Build history of the part. All positions in model axes, mm. Round coordinates to 2 decimals unless told otherwise and drop trailing zeros. Write each loop counter-clockwise with the first axis right and the second up, starting at its lowest first coordinate (ties: lowest second). Pieces come first, ordered by that corner, then holes.
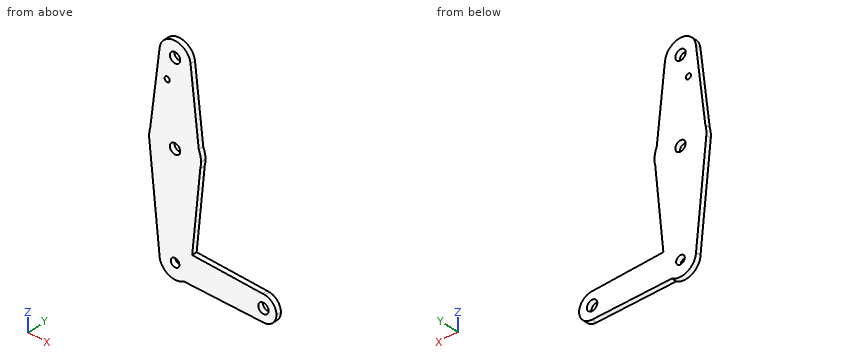
from build123d import *

# Parameters (mm, degrees)
F0_R     = 3.175
F0_R_2   = 2.6335759293
F0_R_3   = 1.5875
F1_DEPTH = 3.048


with BuildPart() as f1:
    # F0 (on Front) → F1 (new body)
    with BuildSketch(Plane.XZ):
        with BuildLine():
            ThreePointArc((56.7990275078, -24.9062731053), (62.4116875835, -22.581433181), (64.7365275078, -16.9687731053))
            ThreePointArc((64.7365275078, -16.9687731053), (62.7426623776, -11.707869116), (57.7627673101, -9.0899970681))
            Line((57.7627673101, -9.0899970681), (56.297547037, -9.0471303724))
            ThreePointArc((56.297547037, -9.0471303724), (48.8654928151, -17.2196386647), (56.7990275078, -24.9062731053))
        make_face()
        with Locations((56.7990275078, -16.9687731053)):
            Circle(F0_R, mode=Mode.SUBTRACT)
        with BuildLine():
            Line((56.297547037, -9.0471303724), (57.7627673101, -9.0899970681))
            ThreePointArc((57.7627673101, -9.0899970681), (57.0311488355, -9.0346678666), (56.297547037, -9.0471303724))
        make_face()
        with BuildLine():
            Line((8.0107625365, -24.9062731053), (56.7990275078, -24.9062731053))
            ThreePointArc((56.7990275078, -24.9062731053), (48.8654928151, -17.2196386647), (56.297547037, -9.0471303724))
            Line((56.297547037, -9.0471303724), (13.2168797338, -7.7867561536))
            Line((13.2168797338, -7.7867561536), (12.2251364065, -17.8985078123))
            ThreePointArc((12.2251364065, -17.8985078123), (10.9082443644, -21.8776629611), (8.0107625365, -24.9062731053))
        make_face()
        with BuildLine():
            ThreePointArc((-6.7763501221, -17.208975122), (-1.652361496, -25.4176415362), (8.0107625365, -24.9062731053))
            ThreePointArc((8.0107625365, -24.9062731053), (10.9082443644, -21.8776629611), (12.2251364065, -17.8985078123))
            ThreePointArc((12.2251364065, -17.8985078123), (12.2592428174, -17.4341964193), (12.2706206818, -16.9687731053))
            ThreePointArc((12.2706206818, -16.9687731053), (9.8779825256, -10.6556883181), (3.9021084446, -7.5142418607))
            ThreePointArc((3.9021084446, -7.5142418607), (-3.6569014681, -9.9165865564), (-6.7763501221, -17.208975122))
        make_face()
        with Locations((2.7456206818, -16.9687731053)):
            Circle(F0_R_2, mode=Mode.SUBTRACT)
        with BuildLine():
            Line((3.9021084446, -7.5142418607), (13.2168797338, -7.7867561536))
            Line((13.2168797338, -7.7867561536), (18.1800145925, 42.8170500531))
            ThreePointArc((18.1800145925, 42.8170500531), (1.6704584717, 30.6926773645), (-13.0491238986, 44.9369657372))
            Line((-13.0491238986, 44.9369657372), (-6.7763501221, -17.208975122))
            ThreePointArc((-6.7763501221, -17.208975122), (-3.6569014681, -9.9165865564), (3.9021084446, -7.5142418607))
        make_face()
        with BuildLine():
            Line((12.2251364065, -17.8985078123), (13.2168797338, -7.7867561536))
            Line((13.2168797338, -7.7867561536), (3.9021084446, -7.5142418607))
            ThreePointArc((3.9021084446, -7.5142418607), (9.8779825256, -10.6556883181), (12.2706206818, -16.9687731053))
            ThreePointArc((12.2706206818, -16.9687731053), (12.2592428174, -17.4341964193), (12.2251364065, -17.8985078123))
        make_face()
        with BuildLine():
            ThreePointArc((-13.0491238986, 44.9369657372), (1.6704584717, 30.6926773645), (18.1800145925, 42.8170500531))
            ThreePointArc((18.1800145925, 42.8170500531), (18.5100843316, 44.6611170492), (18.6206206818, 46.5312268947))
            ThreePointArc((18.6206206818, 46.5312268947), (18.2740618453, 49.830187342), (17.2495164257, 52.9851120231))
            ThreePointArc((17.2495164257, 52.9851120231), (1.7136407932, 62.3726486273), (-12.4730077607, 51.0488560659))
            ThreePointArc((-12.4730077607, 51.0488560659), (-13.0593192868, 48.0210247289), (-13.0491238986, 44.9369657372))
        make_face()
        with Locations((2.7456206818, 46.5312268947)):
            Circle(F0_R, mode=Mode.SUBTRACT)
        with BuildLine():
            Line((-6.7441452961, 98.1497418202), (-12.4730077607, 51.0488560659))
            ThreePointArc((-12.4730077607, 51.0488560659), (1.7136407932, 62.3726486273), (17.2495164257, 52.9851120231))
            Line((17.2495164257, 52.9851120231), (12.2125248757, 98.3816315712))
            ThreePointArc((12.2125248757, 98.3816315712), (12.2560856402, 97.8572319106), (12.2706206818, 97.3312268947))
            ThreePointArc((12.2706206818, 97.3312268947), (2.3359842212, 87.8150394769), (-6.7441452961, 98.1497418202))
        make_face()
        with Locations((-2.1043515299, 83.0673798919)):
            Circle(F0_R_3, mode=Mode.SUBTRACT)
        with BuildLine():
            ThreePointArc((12.2125248757, 98.3816315712), (2.6291136887, 106.8555143284), (-6.7441452961, 98.1497418202))
            ThreePointArc((-6.7441452961, 98.1497418202), (2.3359842212, 87.8150394769), (12.2706206818, 97.3312268947))
            ThreePointArc((12.2706206818, 97.3312268947), (12.2560856402, 97.8572319106), (12.2125248757, 98.3816315712))
        make_face()
        with Locations((2.7456206818, 97.3312268947)):
            Circle(F0_R, mode=Mode.SUBTRACT)
    extrude(amount=F1_DEPTH)


solid = f1.part
1) Slice it at A-A (y = -1.7). Count the separate pieces of the cut face and the enclosed holes in it, plus the area to 3 significant figures.
Results:
separate pieces: 1
enclosed holes: 5
area: 3,890 mm2
2) Pin check, flat tips, straight feed: pin 1 Ø1.5 at (x, y) = (55.5, -2.5) entering from -Z; pin 2 Ø1.5 at (y, z) = (-1, 10) entering from +X. Stop position of each tip, or through.
Results:
pin 1: stops at z = -24.91
pin 2: stops at x = 15.03
3) Slice it at B-B (x = 15). Write the cut outline in (y, z), plus the area to 3 significant figures.
Results:
outline: (-3.05, -24.91) - (0, -24.91) - (0, -7.84) - (-3.05, -7.84) - close; (-3.05, 10.39) - (0, 10.39) - (0, 73.26) - (-3.05, 73.26) - close
area: 244 mm2
4) Slice it at D-D (x = 41.5). Write the cut outline in (y, z), plus the area to 3 significant figures.
Results:
outline: (-3.05, -24.91) - (0, -24.91) - (0, -8.61) - (-3.05, -8.61) - close
area: 49.7 mm2
5) Slice it at C-C (z = 1). Write the cut outline in (x, y).
Results:
outline: (-8.61, -3.05) - (14.08, -3.05) - (14.08, 0) - (-8.61, 0) - close
6) Wall check: L1, parallel to Z at x = 55, y = -0.85; L2, parallel to X at y = -0.3, z = -18.5; L3, parallel to Z at x = -2.5, y = -1.45. Give the ranges that are in metal, low to high.
Results:
L1: z = -24.91 to -19.58, -14.35 to -9.01
L2: x = -6.66 to 0.6, 4.89 to 54.02, 59.58 to 64.59
L3: z = -24.92 to 81.53, 84.6 to 105.28
